from build123d import *

# Parameters (mm, degrees)
SKETCH_1_R      = 11
SKETCH_1_R_2    = 5
SKETCH_1_R_3    = 1.75
EXTRUDE_1_DEPTH = 3.8
EXTRUDE_START   = 1.5
SKETCH_2_R      = 5
SKETCH_2_R_2    = 4
EXTRUDE_2_DEPTH = 15


with BuildPart() as part:
    # 草图1 → 凸台-拉伸1 (new body)
    with BuildSketch(Plane.XY):
        with Locations(Location((0, 0, 0), (0, 0, 180))):
            Circle(SKETCH_1_R)
        with Locations(Location((0, 0, 0), (0, 0, 180))):
            Circle(SKETCH_1_R_2, mode=Mode.SUBTRACT)
        with Locations(Location((-8, 0, 0), (0, 0, 180))):
            Circle(SKETCH_1_R_3, mode=Mode.SUBTRACT)
        with Locations(Location((0, 8, 0), (0, 0, 180))):
            Circle(SKETCH_1_R_3, mode=Mode.SUBTRACT)
        with Locations(Location((8, 0, 0), (0, 0, 180))):
            Circle(SKETCH_1_R_3, mode=Mode.SUBTRACT)
        with Locations(Location((0, -8, 0), (0, 0, 180))):
            Circle(SKETCH_1_R_3, mode=Mode.SUBTRACT)
    extrude(amount=EXTRUDE_1_DEPTH)

    # 草图2 → 凸台-拉伸2 (add)
    with BuildSketch(Plane(origin=(0, 0, 0), x_dir=(-1, 0, 0), z_dir=(0, 0, -1)).offset(EXTRUDE_START)):
        Circle(SKETCH_2_R)
        Circle(SKETCH_2_R_2, mode=Mode.SUBTRACT)
    extrude(amount=-EXTRUDE_2_DEPTH)


solid = part.part
Work out the finished part from the listing and answer in its coordinate system (mm). A direction names the side the tool comes from. Give positions to 0.01 mm unless a question says otherwise; leave off trailing zeros. Loops run counter-clockwise (first coordinate to the right, second up) from the corner with the lowest first, then second, coordinate; pieces in that order, holes last. Notation, with made-up numbers: M 71,53 L 83,53 A23 ccw 83,81 Z; hole C 41,-9.75 d9. An arc over 180 degrees is marked long. Use CSV: the item, a comma, the result in double quotes.
1) Find section A-A on x = 0. Write down the section's boundary in (y, z), plus the area to 3 significant figures.
Answer:
outline,"M -11,0 L -9.75,0 L -9.75,3.8 L -11,3.8 Z; M -6.25,0 L -5,0 L -5,-1.5 L -4,-1.5 L -4,13.5 L -5,13.5 L -5,3.8 L -6.25,3.8 Z; M 4,-1.5 L 5,-1.5 L 5,0 L 6.25,0 L 6.25,3.8 L 5,3.8 L 5,13.5 L 4,13.5 Z; M 9.75,0 L 11,0 L 11,3.8 L 9.75,3.8 Z"
area,"49.0 mm^2"
2) Given P1, Ø4, axis at x = -2.5, z = 8.5, coming from the -Y side; P2, Ø3, axis at x = 5, z = 2.5, coming from the +Y side; P3, Ø8, axis at x = 8.5, y = 6.5, coming from the +Z side; P4, Ø10, axis at x = 6, y = -4, coming from the -Z side, each flat-ended and moving along its own axis, determine where each tip first touches the part or whether it passes through.
Answer:
P1,"y = -4.97"
P2,"y = 10.43"
P3,"z = 3.8"
P4,"z = -1.5"
3) Find section D-D on z = 8.5. Write down the section's boundary in (x, y), plus the area to 3 significant figures.
Answer:
outline,"C 0,0 d10; hole C 0,0 d8"
area,"28.3 mm^2"
4) Consider L1, parallel to Y at x = 0, z = 2; L2, parallel to Y at x = 0, z = 10; L3, parallel to Z at x = -8, y = -5. Determine where each line is inside the solid, lowest interval first.
Answer:
L1,"-11 to -9.75, -6.25 to -4, 4 to 6.25, 9.75 to 11"
L2,"-5 to -4, 4 to 5"
L3,"0 to 3.8"
5) Find section C-C on z = 2.75. Write down the section's boundary in (x, y).
Answer:
outline,"C 0,0 d22; hole C -8,0 d3.5; hole C 0,0 d8; hole C 0,-8 d3.5; hole C 0,8 d3.5; hole C 8,0 d3.5"
6) Determine the mould class of faces 3 (the cylindrical face through (0.867, -3.905, 5.895)), 4 (the cylindrical face through (1.08, -4.88, 8.58)), 5 (the flat face through (-2, 5, 3.8)) for opening direction Y: released by +Y, released by -Y, zero draft, split by the parting line, or undercut.
Answer:
face 3,"undercut"
face 4,"split by the parting line"
face 5,"zero draft"
7) Which of the six approach directions +Z, -Z, +X, -X, +Y, -Y give full straight-line access (tool end or side, diameter ignored) to faces 1 (the cylindrical face through (-0.81, 9.55, 1.87)), 2 (the flat face through (-2, 5, 0))?
Answer:
face 1,"+Z, -Z"
face 2,"-Z"
